Autodesk Inventor part; units mm, degrees
ref_plane "YZ Plane" through (0, 0, 0) normal (1, 0, 0) x (0, 1, 0)
ref_plane "XZ Plane" through (0, 0, 0) normal (0, 1, 0) x (-1, 0, 0)
ref_plane "XY Plane" through (0, 0, 0) normal (0, 0, 1) x (1, 0, 0)
sketch "Sketch2" plane through (0, 0, 0) normal (0, 0, 1) x (1, 0, 0)
  line L0 (0, 0) -> (-9.9, 0)
  line L1 (-4.95, 0) -> (-4.95, 2.5)
  line L2 (-4.95, 0) -> (-2.45, 0) construction
  circle A0 centre (-4.95, 5) radius 2.5
  line L3 (-4.95, 7.5) -> (32.05, 7.5) construction
  line L4 (0, 0) -> (-9.9, 0)
  line L5 (0, 0) -> (-9.9, 0)
  line L6 (-4.95, 7.5) -> (66.05, 7.5) construction
  line L7 (-4.95, 7.5) -> (70.05, 7.5) construction
  line L8 (0, 0) -> (-9.9, 0)
  line L9 (-9.9, 0) -> (-9.9, 82.5)
  line L10 (0, 82.5) -> (0, 0)
  line L11 (0, 82.5) -> (0, 84.5)
  line L12 (0, 84.5) -> (-9.9, 84.5)
  line L13 (-9.9, 84.5) -> (-9.9, 82.5)
  dimension "d35" = 5
  dimension "d33" = 2.5
  dimension "d34" = 90
  dimension "d48" = 9.9
  dimension "d49" = 9.9
  dimension "d50" = 2
extrude "Extrusion6" add sketch "Sketch2" along normal blind 5
properties part number "Cube_Holder_SB_V1_(71mm)"
Check sheet for the modelled part. Datum: model origin and axes. Units: mm. Round coordinates to 2 decimals unless told otherwise and drop trailing zeros. Order: outer loops, then holes, each group sorted by start corner. A loop starts at its lowest first (then second) coordinate and runs counter-clockwise, first axis right, second up.
1) Mould release check, pull along Y, two halves, no side actions. Record for faces 1 (the flat face through (0, 43, 2)), 2 (the cylindrical face through (-2.565, 4.249, 2.465)), 3 (the flat face through (-5, 0, 2)), 4 (the flat face through (-5, 84.5, 2)): +Y half, -Y half, draft (parallel to the pull), parting line (faces both ways), or undercut.
2) Section check C-C (z = 2.35). Record the boundary of the cut face in (x, y).
3) Go/stop test with a flat-tipped pin: pin 1 Ø1 at (y, z) = (57.5, 2.5) entering from +X. Record where the tip stops, or that it passes through.
4) Section check A-A (y = 5). Record the boundary of the cut face in (x, z), and give its area (3 significant figures).
5) Scan lines: line 1 (Y direction, x = -4.95, z = 2.55); line 2 (Y direction, x = -7.25, z = 2.55). Record each from-to range of solid material in increasing order.
6) Section check B-B (x = -4.95). Record the boundary of the cut face in (y, z).
Result:
1. face 1: draft
1. face 2: undercut
1. face 3: -Y half
1. face 4: +Y half
2. outline: (-9.9, 0) - (0, 0) - (0, 84.5) - (-9.9, 84.5) - close; hole circle Ø5 at (-4.95, 5)
3. pin 1: stops at x = 0
4. outline: (-9.9, 0) - (-7.45, 0) - (-7.45, 5) - (-9.9, 5) - close; (-2.45, 0) - (0, 0) - (0, 5) - (-2.45, 5) - close
4. area: 24.5 mm2
5. line 1: y = 0 to 2.5, 7.5 to 84.5
5. line 2: y = 0 to 4.02, 5.98 to 84.5
6. outline: (0, 0) - (2.5, 0) - (2.5, 5) - (0, 5) - close; (7.5, 0) - (84.5, 0) - (84.5, 5) - (7.5, 5) - close
